```python
from build123d import *

# Parameters (mm, degrees)
SKETCH1_W             = 6
SKETCH1_H             = 6
SKETCH1_R             = 1
BOSS_EXTRUDE1_DEPTH   = 15
BOSS_EXTRUDE1_2_DEPTH = 15
BOSS_EXTRUDE1_3_DEPTH = 15
BOSS_EXTRUDE1_4_DEPTH = 15
SKETCH2_W             = 39.5
SKETCH2_H             = 33.999999999
BOSS_EXTRUDE2_DEPTH   = 1
SKETCH3_W             = 39.5
SKETCH3_H             = 33.999999999
BOSS_EXTRUDE3_DEPTH   = 22
SKETCH4_W             = 36.5
SKETCH4_H             = 17.999999999
CUT_EXTRUDE1_DEPTH    = 22
FILLET1_R             = 7
SKETCH7_W             = 6
SKETCH7_H             = 0.6
CUT_EXTRUDE2_DEPTH    = 4
SKETCH8_W             = 9.999999999
SKETCH8_H             = 6
CUT_EXTRUDE3_DEPTH    = 4
FILLET2_R             = 2
SKETCH9_W             = 10
SKETCH9_H             = 6
SKETCH9_W_2           = 9
CUT_EXTRUDE4_DEPTH    = 4
FILLET3_R             = 2
SKETCH10_W            = 10
SKETCH10_H            = 6
CUT_EXTRUDE5_DEPTH    = 4
FILLET4_R             = 2
SKETCH11_W            = 2
SKETCH11_H            = 2
CUT_EXTRUDE6_DEPTH    = 4
SKETCH12_W            = 35.999999999
SKETCH12_H            = 1.5
BOSS_EXTRUDE4_DEPTH   = 65
SKETCH13_W            = 35.999999999
SKETCH13_H            = 1.5
BOSS_EXTRUDE5_DEPTH   = 65
CUT_EXTRUDE7_DEPTH    = 65
CHAMFER1_SIZE         = 10
BOSS_EXTRUDE6_DEPTH   = 1
BOSS_EXTRUDE7_DEPTH   = 1
BOSS_EXTRUDE8_DEPTH   = 1.5
CUT_EXTRUDE8_DEPTH    = 51.5


with BuildPart() as part:
    # Sketch1 → Boss-Extrude1 (new body)
    with BuildSketch(Plane(origin=(0, 0, 0), x_dir=(1, 0, 0), z_dir=(0, 1, 0))):
        with Locations((-7.839776389, 20.365683815)):
            Rectangle(SKETCH1_W, SKETCH1_H)
        with Locations(Location((-7.339776389, 19.865683815, 0), (0, 0, 270))):
            Circle(SKETCH1_R, mode=Mode.SUBTRACT)
    extrude(amount=BOSS_EXTRUDE1_DEPTH)



with BuildPart() as body_2:
    # Sketch1 → Boss-Extrude1 2 (new body)
    with BuildSketch(Plane(origin=(0, 0, 0), x_dir=(1, 0, 0), z_dir=(0, 1, 0))):
        with Locations((25.660223611, 20.365683814)):
            Rectangle(SKETCH1_W, SKETCH1_H)
        with Locations(Location((25.160223611, 19.865683814, 0), (0, 0, 270))):
            Circle(SKETCH1_R, mode=Mode.SUBTRACT)
    extrude(amount=BOSS_EXTRUDE1_2_DEPTH)


with BuildPart() as body_3:
    # Sketch1 → Boss-Extrude1 3 (new body)
    with BuildSketch(Plane(origin=(0, 0, 0), x_dir=(1, 0, 0), z_dir=(0, 1, 0))):
        with Locations((-7.839776389, -7.634316185)):
            Rectangle(SKETCH1_W, SKETCH1_H)
        with Locations(Location((-7.339776389, -7.134316185, 0), (0, 0, 270))):
            Circle(SKETCH1_R, mode=Mode.SUBTRACT)
    extrude(amount=BOSS_EXTRUDE1_3_DEPTH)


with BuildPart() as body_4:
    # Sketch1 → Boss-Extrude1 4 (new body)
    with BuildSketch(Plane(origin=(0, 0, 0), x_dir=(1, 0, 0), z_dir=(0, 1, 0))):
        with Locations((25.660371549, -7.634316185)):
            Rectangle(SKETCH1_W, SKETCH1_H)
        with Locations(Location((25.160371549, -7.134316185, 0), (0, 0, 270))):
            Circle(SKETCH1_R, mode=Mode.SUBTRACT)
    extrude(amount=BOSS_EXTRUDE1_4_DEPTH)


with BuildPart() as part_1:
    add(part.part)

    add(body_2.part)  # Boss-Extrude2 merges body 2

    add(body_3.part)  # Boss-Extrude2 merges body 3

    add(body_4.part)  # Boss-Extrude2 merges body 4
    # Sketch2 → Boss-Extrude2 (add)
    with BuildSketch(Plane.XZ):
        with Locations((8.910223611, -6.365683814)):
            Rectangle(SKETCH2_W, SKETCH2_H)
    extrude(amount=BOSS_EXTRUDE2_DEPTH)

    # Sketch3 → Boss-Extrude3 (add)
    with BuildSketch(Plane.XZ.offset(1)):
        Polygon((-11.839776389, 9.730248223), (-11.839776389, 11.634316185), (29.660223611, 11.634316185), (29.660223611, 9.730248223), (29.660223611, -24.365683814), (28.803720569, -24.365683814), (-10.696279431, -24.365683814), (-11.839776389, -24.365683814), align=None)
        with Locations((8.910223611, -6.365683814)):
            Rectangle(SKETCH3_W, SKETCH3_H, mode=Mode.SUBTRACT)
    extrude(amount=-BOSS_EXTRUDE3_DEPTH)

    # Sketch4 → Cut-Extrude1 (cut)
    with BuildSketch(Plane(origin=(0, 0, 0), x_dir=(1, 0, 0), z_dir=(0, 1, 0))):
        with Locations((10.410223611, 6.365683815)):
            Rectangle(SKETCH4_W, SKETCH4_H)
    extrude(amount=-CUT_EXTRUDE1_DEPTH, mode=Mode.SUBTRACT)

    # Fillet1
    fillet1_edges = [part_1.edges().sort_by_distance(p)[0] for p in [
        (-7.839776389, -0.5, 2.634316185),
        (-7.839776389, -0.5, -15.365683814),
        (28.660223611, -0.5, -15.365683814),
        (28.660223611, -0.5, 2.634316185),
    ]]
    fillet(fillet1_edges, radius=FILLET1_R)

    # Sketch7 → Cut-Extrude2 (cut)
    with BuildSketch(Plane(origin=(0, 15, 0), x_dir=(1, 0, 0), z_dir=(0, 1, 0))):
        with Locations((-7.839776389, 17.665683815)):
            Rectangle(SKETCH7_W, SKETCH7_H)
        with Locations((-7.839776389, -4.934316185)):
            Rectangle(SKETCH7_W, SKETCH7_H)
    extrude(amount=-CUT_EXTRUDE2_DEPTH, mode=Mode.SUBTRACT)

    # Sketch8 → Cut-Extrude3 (cut)
    with BuildSketch(Plane.ZY.offset(-28.660223611)):
        with Locations((-6.365683815, 18)):
            Rectangle(SKETCH8_W, SKETCH8_H)
    extrude(amount=-CUT_EXTRUDE3_DEPTH, mode=Mode.SUBTRACT)

    # Fillet2
    fillet2_edges = [part_1.edges().sort_by_distance(p)[0] for p in [
        (29.160223611, 15, -11.365683814),
        (29.160223611, 15, -1.365683815),
    ]]
    fillet(fillet2_edges, radius=FILLET2_R)

    # Sketch9 → Cut-Extrude4 (cut)
    with BuildSketch(Plane(origin=(0, 0, 10.634316185), x_dir=(-1, 0, 0), z_dir=(0, 0, -1))):
        with Locations((-14.660371549, 18)):
            Rectangle(SKETCH9_W, SKETCH9_H)
        with Locations((-0.660223611, 18)):
            Rectangle(SKETCH9_W_2, SKETCH9_H)
    extrude(amount=-CUT_EXTRUDE4_DEPTH, mode=Mode.SUBTRACT)

    # Fillet3
    fillet3_edges = [part_1.edges().sort_by_distance(p)[0] for p in [
        (19.660371549, 15, 11.134316185),
        (9.660371549, 15, 11.134316185),
        (5.160223611, 15, 11.134316185),
        (-3.839776389, 15, 11.134316185),
    ]]
    fillet(fillet3_edges, radius=FILLET3_R)

    # Sketch10 → Cut-Extrude5 (cut)
    with BuildSketch(Plane.XY.offset(-23.365683814)):
        with Locations((14.660223611, 18)):
            Rectangle(SKETCH10_W, SKETCH10_H)
    extrude(amount=-CUT_EXTRUDE5_DEPTH, mode=Mode.SUBTRACT)

    # Fillet4
    fillet4_edges = [part_1.edges().sort_by_distance(p)[0] for p in [
        (19.660223611, 15, -23.865683814),
        (9.660223611, 15, -23.865683814),
    ]]
    fillet(fillet4_edges, radius=FILLET4_R)

    # Sketch11 → Cut-Extrude6 (cut)
    with BuildSketch(Plane.XY.offset(-23.365683814)):
        with Locations((0.160223611, 17)):
            Rectangle(SKETCH11_W, SKETCH11_H)
    extrude(amount=-CUT_EXTRUDE6_DEPTH, mode=Mode.SUBTRACT)

    # Sketch12 → Boss-Extrude4 (add)
    with BuildSketch(Plane.ZY.offset(11.839776389)):
        with Locations((-6.365683814, -0.25)):
            Rectangle(SKETCH12_W, SKETCH12_H)
    extrude(amount=BOSS_EXTRUDE4_DEPTH)

    # Sketch13 → Boss-Extrude5 (add)
    with BuildSketch(Plane(origin=(29.660223611, 0, 0), x_dir=(0, 0, -1), z_dir=(1, 0, 0))):
        with Locations((6.365683814, -0.25)):
            Rectangle(SKETCH13_W, SKETCH13_H)
    extrude(amount=BOSS_EXTRUDE5_DEPTH)

    # Sketch14 → Cut-Extrude7 (cut)
    with BuildSketch(Plane(origin=(0, 0.5, 0), x_dir=(1, 0, 0), z_dir=(0, 1, 0))):
        with BuildLine():
            Line((-68.539776389, 8.115683814), (-66.789776389, 8.115683814))
            ThreePointArc((-66.789776389, 8.115683814), (-65.039776389, 6.365683814), (-66.789776389, 4.615683814))
            Line((-66.789776389, 4.615683814), (-68.539776389, 4.615683814))
            ThreePointArc((-68.539776389, 4.615683814), (-70.289776389, 6.365683814), (-68.539776389, 8.115683814))
        make_face()
        with BuildLine():
            Line((84.610223611, 8.115683814), (86.360223611, 8.115683814))
            ThreePointArc((86.360223611, 8.115683814), (88.110223611, 6.365683814), (86.360223611, 4.615683814))
            Line((86.360223611, 4.615683814), (84.610223611, 4.615683814))
            ThreePointArc((84.610223611, 4.615683814), (82.860223611, 6.365683814), (84.610223611, 8.115683814))
        make_face()
    extrude(amount=-CUT_EXTRUDE7_DEPTH, mode=Mode.SUBTRACT)

    # Chamfer1
    chamfer1_edges = [part_1.edges().sort_by_distance(p)[0] for p in [
        (-76.839776389, -0.25, -24.365683814),
        (-76.839776389, -0.25, 11.634316185),
        (94.660223611, -0.25, 11.634316185),
        (94.660223611, -0.25, -24.365683814),
    ]]
    chamfer(chamfer1_edges, length=CHAMFER1_SIZE)

    # Sketch15 → Boss-Extrude6 (add)
    with BuildSketch(Plane.XY.offset(11.634316185)):
        Polygon((-66.839776389, 0.5), (-11.839776389, 10.75), (-11.839776389, 0.5), align=None)
        Polygon((29.660223611, 10.75), (84.660223611, 0.5), (29.660223611, 0.5), align=None)
    extrude(amount=-BOSS_EXTRUDE6_DEPTH)

    # Sketch16 → Boss-Extrude7 (add)
    with BuildSketch(Plane(origin=(0, 0, -24.365683814), x_dir=(-1, 0, 0), z_dir=(0, 0, -1))):
        Polygon((-29.660223611, 10.75), (-84.660223611, 0.5), (-29.660223611, 0.5), align=None)
        Polygon((11.839776389, 10.75), (66.839776389, 0.5), (11.839776389, 0.5), align=None)
    extrude(amount=-BOSS_EXTRUDE7_DEPTH)

    # Sketch17 → Boss-Extrude8 (add)
    with BuildSketch(Plane(origin=(0, 0.5, 0), x_dir=(1, 0, 0), z_dir=(0, 1, 0))):
        Polygon((-11.839776389, 23.365683814), (-37.622747474, 6.958338579), (-64.97714713, 24.365683814), (-66.839776389, 24.365683814), (-38.554062103, 6.365683814), (-66.839776389, -11.634316185), (-64.97714713, -11.634316185), (-37.622747474, 5.77302905), (-11.839776389, -10.634316185), (-11.839776389, -9.449006657), (-36.691432844, 6.365683814), (-11.839776389, 22.180374286), align=None)
        Polygon((29.660223611, 23.365683814), (55.443194696, 6.958338579), (82.797594352, 24.365683814), (84.660223611, 24.365683814), (56.374509325, 6.365683814), (84.660223611, -11.634316185), (82.797594352, -11.634316185), (55.443194696, 5.77302905), (29.660223611, -10.634316185), (29.660223611, -9.449006657), (54.511880067, 6.365683814), (29.660223611, 22.180374286), align=None)
    extrude(amount=BOSS_EXTRUDE8_DEPTH)

    # Sketch18 → Cut-Extrude8 (cut)
    with BuildSketch(Plane.XY.offset(11.634316185)):
        Polygon((-57.576355355, 2.226364829), (-66.839776389, 0.5), (-66.839776389, 4.287768192), align=None)
        Polygon((75.79220332, 2.152676509), (84.660223611, 0.5), (84.660223611, 4.287768192), align=None)
    extrude(amount=-CUT_EXTRUDE8_DEPTH, mode=Mode.SUBTRACT)


solid = part_1.part
```
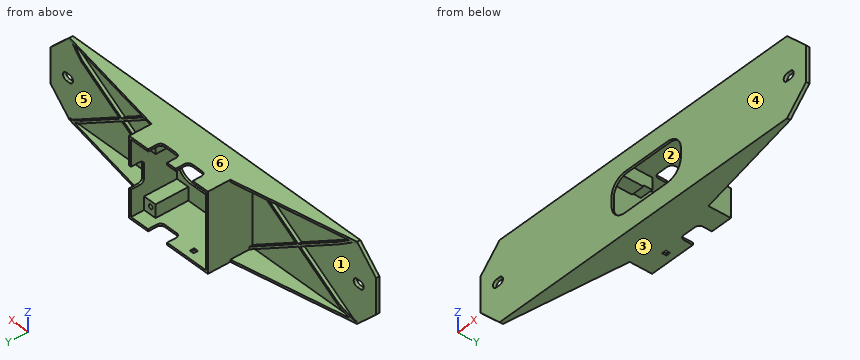
Check sheet for the modelled part. Datum: model origin and axes. Units: mm. Face numbers are marked on the shaded views. A direction names the side the tool comes from. Round coordinates to 2 decimals unless told otherwise and drop trailing zeros. Write each loop counter-clockwise with the first axis right and the second up, starting at its lowest first coordinate (ties: lowest second). Pieces come first, ordered by that corner, then holes. Notation, with made-up numbers: (56.25, 55) -> (71.25, 55) arc R24 cw to (71.25, 68) -> close; hole circle Ø11 at (64.25, -7). An arc over 180 degrees is marked (long way). One line per question, with ' | ' between items. Start each with the question number.
1. Sectioned sample at C-C, the plane x = -18. Record the cut outline in (y, z), then the cut area to 3 significant figures.
2. Sectioned sample at A-A, the plane y = 4.25. Record the cut outline in (x, z), then the cut area to 3 significant figures.
3. Release check for a two-part mould opening along Z. For the marked faces 3, 4, 5 and 6 record: +Z half, -Z half, draft (parallel to the pull), parting line (faces both ways), or undercut.
4. Depth check by flat-ended pin: pin 1 (3 mm diameter, centred on y = 9.5, z = 7.5, fed in from +X); pin 2 (7.5 mm diameter, centred on x = -23.5, z = -13, fed in from +Y); pin 3 (1.5 mm diameter, centred on y = 18.5, z = 1.5, fed in from -X). Enter the tip coordinate at first touch or a pass-through.
5. Set-up check for the marked faces 1 and 2: record each of +Z, -Z, +X, -X, +Y, -Y from which the full face is reachable in a straight line by a thin tool's end or side.
6. Scan lines: line 1 along Z through (x, y) = (17, 1); line 2 along X through (y, z) = (11.75, 6); line 3 along X through (y, z) = (17.5, 9.5). Record each from-to range of solid material in increasing order. Write a range as from..to.
7. Sectioned sample at B-B, the plane x = 64. Record the cut outline in (y, z), then the cut area to 3 significant figures.
Taken from the geometry:
1) outline: (-1, -24.37) -> (9.6, -24.37) -> (9.6, -23.37) -> (0.5, -23.37) -> (0.5, -19.45) -> (2, -19.45) -> (2, -18.26) -> (0.5, -18.26) -> (0.5, 5.53) -> (2, 5.53) -> (2, 6.71) -> (0.5, 6.71) -> (0.5, 10.63) -> (9.6, 10.63) -> (9.6, 11.63) -> (-1, 11.63) -> close | area: 75.8 mm^2
2) outline: (-46.72, -24.37) -> (64.54, -24.37) -> (64.54, -23.37) -> (29.66, -23.37) -> (29.66, 10.63) -> (64.54, 10.63) -> (64.54, 11.63) -> (-46.72, 11.63) -> (-46.72, 10.63) -> (-11.84, 10.63) -> (-11.84, -23.37) -> (-46.72, -23.37) -> close; hole (-10.84, -17.37) -> (-4.84, -17.37) -> (-4.84, -23.37) -> (22.66, -23.37) -> (22.66, -17.37) -> (28.66, -17.37) -> (28.66, 4.63) -> (22.66, 4.63) -> (22.66, 10.63) -> (-4.84, 10.63) -> (-4.84, 4.63) -> (-10.84, 4.63) -> close; hole circle Ø2 at (-7.34, -19.87); hole circle Ø2 at (-7.34, 7.13); hole circle Ø2 at (25.16, -19.87); hole circle Ø2 at (25.16, 7.13) | area: 422 mm^2
3) face 3: -Z half | face 4: draft | face 5: undercut | face 6: +Z half
4) pin 1: stops at x = 29.66 | pin 2: stops at y = 2 | pin 3: stops at x = -11.84
5) face 1: -X, +Y | face 2: +Y
6) line 1: z = -24.37..-23.37, 10.63..11.63 | line 2: x = -11.84..-4.84, 22.66..29.66 | line 3: x = -11.84..-10.84, 28.66..29.66
7) outline: (-1, -24.37) -> (4.35, -24.37) -> (4.35, -23.37) -> (0.5, -23.37) -> (0.5, -12.4) -> (2, -12.4) -> (2, -11.22) -> (0.5, -11.22) -> (0.5, -1.51) -> (2, -1.51) -> (2, -0.33) -> (0.5, -0.33) -> (0.5, 10.63) -> (4.35, 10.63) -> (4.35, 11.63) -> (-1, 11.63) -> close | area: 65.3 mm^2
